For this review, use the dimensioned drawing (mm, ordinates from the lowest corner) and the shaded views. Give positions to 0.01 mm unless a question says otherwise; leave off trailing zeros. Write each loop counter-clockwise with the first axis right and the second up, starting at its lowest first coordinate (ties: lowest second). Pieces come first, ordered by that corner, then holes. Notation, with made-up numbers: M 46.5,-25 L 64.5,-25 A26 ccw 64.5,-10 Z; hole C -31.5,48.25 d2. An arc over 180 degrees is marked long. Answer in a Markdown table with one row per item.
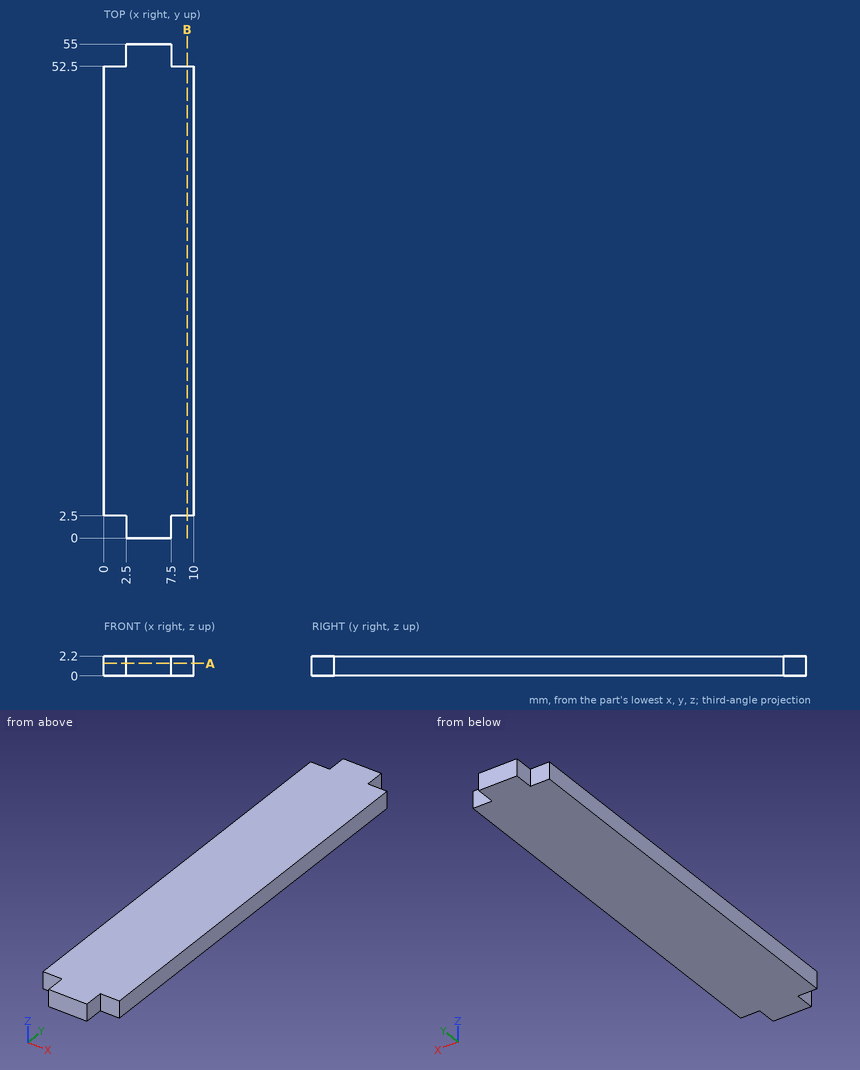
1) Add section A-A (z = 1.4). Write out the cut boundary in (x, y).
Geometry says:
| item | result |
|---|---|
| outline | M 0,2.5 L 2.5,2.5 L 2.5,0 L 7.5,0 L 7.5,2.5 L 10,2.5 L 10,52.5 L 7.5,52.5 L 7.5,55 L 2.5,55 L 2.5,52.5 L 0,52.5 Z |
2) Add section B-B (x = 9.25). Write out the cut boundary in (y, z), and give its area (3 significant figures).
Geometry says:
| item | result |
|---|---|
| outline | M 2.5,0 L 52.5,0 L 52.5,2.2 L 2.5,2.2 Z |
| area | 110 mm^2 |
3) To check wall thickness, follow probe 1 along Y at (x, z) = (1, 1.35). State the ranges of the line that lie inside material, in increasing order. Write a range as [from, to].
Geometry says:
| item | result |
|---|---|
| probe 1 | [2.5, 52.5] |
4) Insertion check: P1, Ø1.1, axis at x = 1, z = 0.5, coming from the -Y side; P2, Ø1.1, axis at y = 53.5, z = 1.5, coming from the -X side; P3, Ø1.1, axis at y = 0.5, z = 1, coming from the +X side. Each pin has a flat end and moves straight along its axis. Give the tip position at first contact, or say it passes through.
Geometry says:
| item | result |
|---|---|
| P1 | y = 2.5 |
| P2 | x = 2.5 |
| P3 | x = 7.5 |
